```python
from build123d import *

# Parameters (mm, degrees)
SKETCH1_R               = 20
BOSS_EXTRUDE1_DEPTH     = 590
SKETCH2_R               = 18
CUT_EXTRUDE1_DEPTH      = 602
CUT_EXTRUDE2_DEPTH      = 591.677577025
CUT_EXTRUDE2_DEPTH_BACK = 591.677577025
SKETCH3_R               = 5


with BuildPart() as part:
    # Sketch1 → Boss-Extrude1 (new body)
    with BuildSketch(Plane(origin=(0, 0, 0), x_dir=(0, 0, -1), z_dir=(1, 0, 0))):
        Circle(SKETCH1_R)
    extrude(amount=BOSS_EXTRUDE1_DEPTH)

    # Sketch2 → Cut-Extrude1 (cut)
    with BuildSketch(Plane(origin=(590, 0, 0), x_dir=(0, 0, -1), z_dir=(1, 0, 0))):
        Circle(SKETCH2_R)
    extrude(amount=-CUT_EXTRUDE1_DEPTH, mode=Mode.SUBTRACT)

    # Sketch3 → Cut-Extrude2 (cut, two sides: drawn at the far end of the back side and taken through both)
    with BuildSketch(Plane.XY.offset(-CUT_EXTRUDE2_DEPTH_BACK)):
        with Locations((154.855292025, 0)):
            Circle(SKETCH3_R)
        with Locations((354.855292025, 0)):
            Circle(SKETCH3_R)
    extrude(amount=CUT_EXTRUDE2_DEPTH + CUT_EXTRUDE2_DEPTH_BACK, mode=Mode.SUBTRACT)


solid = part.part
```
The model under review builds one solid part; all positions refer to its coordinate system, in mm. Round coordinates to 2 decimals unless told otherwise and drop trailing zeros. Loops run counter-clockwise (first coordinate to the right, second up) from the corner with the lowest first, then second, coordinate; pieces in that order, holes last. Notation, with made-up numbers: M 68.25,-6 L 77.25,-6 A20 cw 77.25,25 Z; hole C 47.25,-7 d3. An arc over 180 degrees is marked long. Answer as a JSON object with one key per item and string values.
(1) To check wall thickness, follow line 1 along X through (y, z) = (0, -19); line 2 along Y through (x, z) = (391, 0). State the ranges of each line that lie inside material, in increasing order.
Resolved:
{"line 1": "0 to 149.86, 159.86 to 349.86, 359.86 to 590", "line 2": "-20 to -18, 18 to 20"}
(2) Clearance check with flat-ended pins moving along their axes: P1, Ø13, axis at x = 354.86, y = 0, coming from the -Z side; P2, Ø2, axis at x = 195.5, z = -12.5, coming from the +Y side; P3, Ø9, axis at x = 354.86, y = 0, coming from the -Z side (3 decimals); P4, Ø12, axis at x = 491, y = 13, coming from the +Z side (3 decimals). State where each tip first meets the part, or that it passes through.
Resolved:
{"P1": "z = -20", "P2": "y = 16.36", "P3": "through", "P4": "z = 18.735"}
(3) Draft analysis for pull direction Z (two halves, no side actions). For faces 1 (the cylindrical face through (290.87, 6.007, -19.076)), 2 (the cylindrical face through (299.13, 17.847, 2.343)), 3 (the flat face through (0, 3, 18)), state which applies: released by +Z, released by -Z, zero draft, split by the parting line, or undercut.
Resolved:
{"face 1": "split by the parting line", "face 2": "undercut", "face 3": "zero draft"}
(4) Take a section at C-C on x = 70. Give the boundary of the cut face in (y, z), and give its area (3 significant figures).
Resolved:
{"outline": "C 0,0 d40; hole C 0,0 d36", "area": "239 mm²"}
(5) Take a section at B-B on z = 0. Give the boundary of the cut face in (x, y), and give its area (3 significant figures).
Resolved:
{"outline": "M 0,-20 L 590,-20 L 590,-18 L 0,-18 Z; M 0,18 L 590,18 L 590,20 L 0,20 Z", "area": "2,360 mm²"}
(6) Take a section at A-A on y = 0. Give the boundary of the cut face in (x, z), and give its area (3 significant figures).
Resolved:
{"outline": "M 0,-20 L 149.86,-20 L 149.86,-18 L 0,-18 Z; M 0,18 L 149.86,18 L 149.86,20 L 0,20 Z; M 159.86,-20 L 349.86,-20 L 349.86,-18 L 159.86,-18 Z; M 159.86,18 L 349.86,18 L 349.86,20 L 159.86,20 Z; M 359.86,-20 L 590,-20 L 590,-18 L 359.86,-18 Z; M 359.86,18 L 590,18 L 590,20 L 359.86,20 Z", "area": "2,280 mm²"}
